Read the model definition and answer for the solid it produces. Units are mm, in the model's axes. Face numbers are marked on the shaded views. A direction names the side the tool comes from. Coordinates: 2 decimals unless noted, no trailing zeros. Order: outer loops, then holes, each group sorted by start corner. A loop starts at its lowest first (then second) coordinate and runs counter-clockwise, first axis right, second up. Notation, with made-up numbers: M 65.25,65.5 L 99.25,65.5 A18 ccw 99.25,90.5 Z; hole C 85.25,-20 d1. An arc over 180 degrees is marked long. Use a Markdown table: item, result. Add a question column.
1) Find section C-C on x = -27. Write down the section's boundary in (y, z).
2) Find section A-A on z = 5.25. Write down the section's boundary in (x, y).
3) For the marked faces 1 and 2, determine the directions among +Z, -Z, +X, -X, +Y, -Y from which every point of the face is accessible in a straight line to the end or side of a thin tool.
4) Find the intervals of material crossed by probe 1 along Y at (x, z) = (-0.5, 7.5); probe 2 along X at (y, z) = (-21, 7.5); probe 3 along X at (y, z) = (28, 8), in increasing order. Write a range as [from, to].
5) Find section B-B on y = 23. Write down the section's boundary in (x, z), plus the area to 3 significant figures.
6) The mould has two halves that part along X. Classify the marked faces 3, 4 and 5: released by +X, released by -X, zero draft, split by the parting line, or undercut.
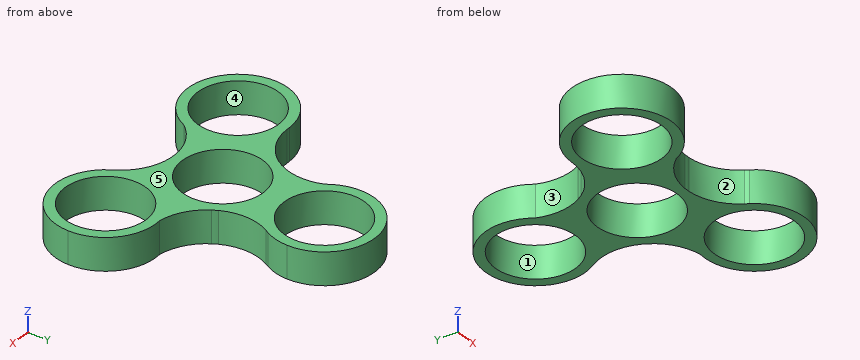
from build123d import *

# Parameters (mm, degrees)
F0_R     = 11.25
F1_DEPTH = 9


with BuildPart() as f1:
    # F0 (on Top) → F1 (new body)
    with BuildSketch(Plane.XY):
        with BuildLine():
            ThreePointArc((0.7608400883, -13.9793105109), (10.1649338718, -9.6267398107), (14, 0))
            ThreePointArc((14, 0), (13.6288181517, 3.2023921975), (12.5349548876, 6.2349744158))
            ThreePointArc((12.5349548876, 6.2349744158), (12.110837047, 6.930523737), (11.7260179857, 7.6485621001))
            ThreePointArc((11.7260179857, 7.6485621001), (0.0535862893, 13.9998974464), (-11.6671236798, 7.73810216))
            ThreePointArc((-11.6671236798, 7.73810216), (-12.0574281413, 7.0230306753), (-12.486858074, 6.3307484108))
            ThreePointArc((-12.486858074, 6.3307484108), (-12.1510599836, -6.9535416354), (-0.8678312078, -13.9730765759))
            ThreePointArc((-0.8678312078, -13.9730765759), (-0.0534089057, -13.9535544123), (0.7608400883, -13.9793105109))
        make_face()
        Circle(F0_R, mode=Mode.SUBTRACT)
        with BuildLine():
            ThreePointArc((12.5349548876, 6.2349744158), (13.6288181517, 3.2023921975), (14, 0))
            ThreePointArc((14, 0), (10.1649338718, -9.6267398107), (0.7608400883, -13.9793105109))
            ThreePointArc((0.7608400883, -13.9793105109), (7.352091686, -15.9948371419), (12.2933676324, -20.8001193652))
            ThreePointArc((12.2933676324, -20.8001193652), (12.2592417259, -7.7393660933), (23.0177448502, -0.3340267271))
            ThreePointArc((23.0177448502, -0.3340267271), (17.0493592663, 1.7903446823), (12.5349548876, 6.2349744158))
        make_face()
        with BuildLine():
            ThreePointArc((11.7260179857, 7.6485621001), (12.110837047, 6.930523737), (12.5349548876, 6.2349744158))
            ThreePointArc((12.5349548876, 6.2349744158), (12.1510599836, 6.9535416354), (11.7260179857, 7.6485621001))
        make_face()
        with BuildLine():
            ThreePointArc((-0.8678312078, -13.9730765759), (-0.0535862893, -13.9998974464), (0.7608400883, -13.9793105109))
            ThreePointArc((0.7608400883, -13.9793105109), (-0.0534089057, -13.9535544123), (-0.8678312078, -13.9730765759))
        make_face()
        with BuildLine():
            ThreePointArc((-11.6671236798, 7.73810216), (0.0535862893, 13.9998974464), (11.7260179857, 7.6485621001))
            ThreePointArc((11.7260179857, 7.6485621001), (10.1758894553, 14.3645171298), (11.8667483176, 21.0464290365))
            ThreePointArc((11.8667483176, 21.0464290365), (0.5728671472, 14.4864978581), (-11.2195968121, 20.1009651281))
            ThreePointArc((-11.2195967939, 20.1009651416), (-10.0751636095, 13.8700059017), (-11.6671236798, 7.73810216))
        make_face()
        with BuildLine():
            ThreePointArc((38.6598761714, -14.2373862032), (33.9606869292, -3.7734042055), (23.0177448502, -0.3340267271))
            ThreePointArc((23.0177448502, -0.3340267271), (12.2592417259, -7.7393660933), (12.2933676324, -20.8001193652))
            ThreePointArc((12.2933676324, -20.8001193652), (12.5679698707, -21.254196273), (12.8259555181, -21.7179156204))
            ThreePointArc((12.8259554695, -21.7179156511), (28.5537887393, -27.6849675811), (38.6598761714, -14.2373862032))
        make_face()
        with Locations((24.6598761714, -14.2373862032)):
            Circle(F0_R, mode=Mode.SUBTRACT)
        with BuildLine():
            ThreePointArc((-11.7981480563, -19.7669384146), (-6.9741956568, -15.660350584), (-0.8678312078, -13.9730765759))
            ThreePointArc((-0.8678312078, -13.9730765759), (-12.1510599836, -6.9535416354), (-12.486858074, 6.3307484108))
            ThreePointArc((-12.486858074, 6.3307484108), (-17.5279813167, 1.6303202988), (-24.1601159998, -0.246309001))
            ThreePointArc((-24.1601159998, -0.246309001), (-14.5852387143, -4.5161887863), (-10.659876271, -14.2373861458))
            ThreePointArc((-10.659876271, -14.2373861458), (-10.9473966527, -17.0601335163), (-11.7981480879, -19.766938401))
        make_face()
        with BuildLine():
            ThreePointArc((12.8259555181, -21.7179156204), (12.5679698707, -21.254196273), (12.2933676324, -20.8001193652))
            ThreePointArc((12.2933676324, -20.8001193652), (12.550962869, -21.2640652647), (12.8259554695, -21.7179156511))
        make_face()
        with BuildLine():
            ThreePointArc((-12.486858074, 6.3307484108), (-12.0574281413, 7.0230306753), (-11.6671236798, 7.73810216))
            ThreePointArc((-11.6671236798, 7.73810216), (-12.0974736943, 7.046355811), (-12.486858074, 6.3307484108))
        make_face()
        with BuildLine():
            ThreePointArc((12.3952888855, 21.9665611167), (12.1226891672, 21.5112796549), (11.8667483176, 21.0464290365))
            ThreePointArc((11.8667483176, 21.0464290365), (12.1397394153, 21.5014856829), (12.3952888855, 21.9665611167))
        make_face()
        with BuildLine():
            ThreePointArc((-11.2195968121, 20.1009651281), (0.5728671472, 14.4864978581), (11.8667483176, 21.0464290365))
            ThreePointArc((11.8667483176, 21.0464290365), (12.1226891672, 21.5112796549), (12.3952888855, 21.9665611167))
            ThreePointArc((12.3952888855, 21.9665611167), (13.5929033763, 25.1232088629), (14, 28.474772349))
            ThreePointArc((14, 28.474772349), (-4.4116688809, 41.7615017315), (-11.2195968121, 20.1009651281))
        make_face()
        with Locations((0, 28.474772349)):
            Circle(F0_R, mode=Mode.SUBTRACT)
        with BuildLine():
            ThreePointArc((-25.2212444048, -0.2486454655), (-36.1952849813, -22.1705031804), (-11.7981480879, -19.766938401))
            ThreePointArc((-11.7981480879, -19.766938401), (-10.9473966527, -17.0601335163), (-10.659876271, -14.2373861458))
            ThreePointArc((-10.659876271, -14.2373861458), (-14.5852387143, -4.5161887863), (-24.1601159998, -0.246309001))
            ThreePointArc((-24.1601159998, -0.246309001), (-24.6906590507, -0.257083046), (-25.2212444036, -0.2486454962))
        make_face()
        with Locations((-24.659876271, -14.2373861458)):
            Circle(F0_R, mode=Mode.SUBTRACT)
        with BuildLine():
            ThreePointArc((-25.2212444036, -0.2486454962), (-24.6906590507, -0.257083046), (-24.1601159998, -0.246309001))
            ThreePointArc((-24.1601159998, -0.246309001), (-24.6907023468, -0.2374200832), (-25.2212444048, -0.2486454655))
        make_face()
    extrude(amount=F1_DEPTH)


solid = f1.part
Check result:
| question | item | result |
|---|---|---|
| 1 | outline | M -28.04,0 L -25.24,0 L -25.24,9 L -28.04,9 Z; M -3.23,0 L -0.43,0 L -0.43,9 L -3.23,9 Z |
| 2 | outline | M -24.16,-0.25 A14 ccw long -11.8,-19.77 A14.66 cw -0.87,-13.97 A14 ccw 0.76,-13.98 A14.66 cw 12.29,-20.8 A14 ccw long 23.02,-0.33 A14.66 cw 12.53,6.23 A14 ccw 11.73,7.65 A14.66 cw 11.87,21.05 A14 ccw long -11.22,20.1 A14.66 cw -11.67,7.74 A14 ccw -12.49,6.33 A14.66 cw Z; hole C -24.66,-14.24 d22.5; hole C 0,0 d22.5; hole C 0,28.47 d22.5; hole C 24.66,-14.24 d22.5 |
| 3 | face 1 | +Z, -Z |
| 3 | face 2 | +Z, -Z, -Y |
| 4 | probe 1 | y = [-13.99, -11.24], [11.24, 17.24], [39.71, 42.47] |
| 4 | probe 2 | x = [-36.92, -33.65], [-15.67, -12.4], [12.4, 15.67], [33.65, 36.92] |
| 4 | probe 3 | x = [-13.99, -11.24], [11.24, 13.99] |
| 5 | outline | M -12.89,0 L -9.83,0 L -9.83,9 L -12.89,9 Z; M 9.83,0 L 12.89,0 L 12.89,9 L 9.83,9 Z |
| 5 | area | 55.0 mm2 |
| 6 | face 3 | released by -X |
| 6 | face 4 | undercut |
| 6 | face 5 | zero draft |
